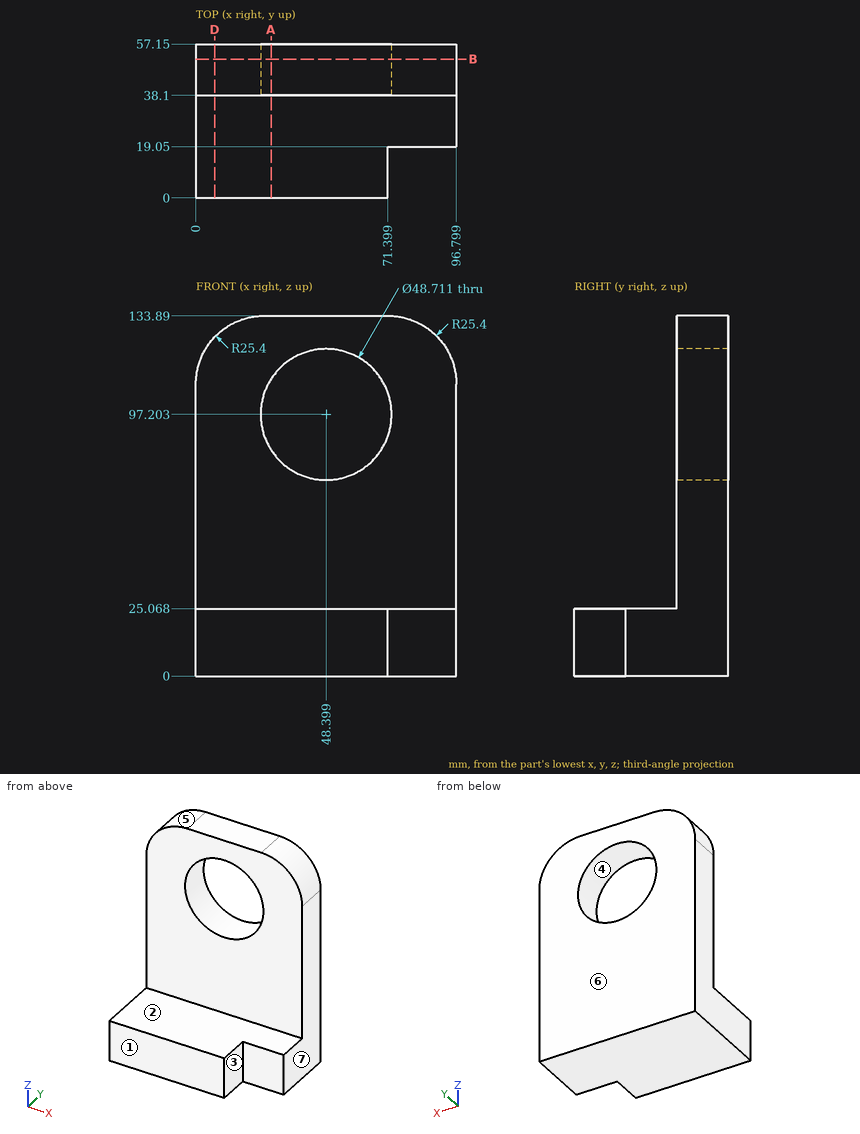
Part print with two shaded views. Sizes in mm from the minimum x, y, z corner. A direction names the side the tool comes from. Round coordinates to 2 decimals unless told otherwise and drop trailing zeros. Order: outer loops, then holes, each group sorted by start corner. A loop starts at its lowest first (then second) coordinate and runs counter-clockwise, first axis right, second up. Notation, with made-up numbers: (66.5, 35) - (123.5, 35) arc R5 cw to (123.5, 40) - close; hole circle Ø11 at (80.5, 29.25). An arc over 180 degrees is marked (long way). Return JSON: item names as keys, results as strings.
(1) Tool access for the marked faces 1, 2 and 3: list every direction of +Z, -Z, +X, -X, +Y, -Y with a clear straight run to the whole face (end or side of a thin tool).
Answer key:
{"face 1": "+Z, -Z, +X, -X, -Y", "face 2": "+Z, +X, -X, -Y", "face 3": "+Z, -Z, +X, -Y"}
(2) Cut at D-D (x = 7). Give the cut face in (y, z), then the cut area to 3 significant figures.
Answer key:
{"outline": "(0, 0) - (57.15, 0) - (57.15, 126) - (38.1, 126) - (38.1, 25.07) - (0, 25.07) - close", "area": "3,360 mm^2"}
(3) Cut at B-B (y = 51.5). Give the cut face in (x, z) (1 decimal).
Answer key:
{"outline": "(0, 0) - (96.8, 0) - (96.8, 108.5) arc R25.4 ccw to (71.4, 133.9) - (25.4, 133.9) arc R25.4 ccw to (0, 108.5) - close; hole circle Ø48.7 at (48.4, 97.2)"}
(4) Cut at A-A (x = 28). Give the cut face in (y, z), then the cut area to 3 significant figures.
Answer key:
{"outline": "(0, 0) - (57.15, 0) - (57.15, 83.9) - (38.1, 83.9) - (38.1, 25.07) - (0, 25.07) - close; (38.1, 110.51) - (57.15, 110.51) - (57.15, 133.89) - (38.1, 133.89) - close", "area": "3,000 mm^2"}
(5) Wall check: probe 1 along X at (y, z) = (39, 97.5) (1 decimal); probe 2 along Y at (x, z) = (85.5, 49); probe 3 along Z at (x, y) = (21, 35). Give the ranges that are in metal, low to high. Write a range as from..to.
Answer key:
{"probe 1": "x = 0..24, 72.8..96.8", "probe 2": "y = 38.1..57.15", "probe 3": "z = 0..25.07"}
(6) Pull direction X, two halves, no side cores. Call the marked faces 4, 5, 6 and 7: +X half, -X half, draft (parallel to the pull), parting line (faces both ways), or undercut.
Answer key:
{"face 4": "undercut", "face 5": "-X half", "face 6": "draft", "face 7": "+X half"}
(7) Pin check, flat tips, straight feed: pin 1 Ø1.5 at (x, y) = (14.5, 43) entering from +Z; pin 2 Ø9.5 at (y, z) = (7.5, 16) entering from +X; pin 3 Ø1 at (x, y) = (42.5, 7.5) entering from +Z. Stop position of each tip, or through.
Answer key:
{"pin 1": "stops at z = 131.77", "pin 2": "stops at x = 71.4", "pin 3": "stops at z = 25.07"}
